Source: CAD feature listing. Evaluate the final solid. Frame: model axes, mm. A direction names the side the tool comes from. Coordinates: 2 decimals unless noted, no trailing zeros. Order: outer loops, then holes, each group sorted by start corner. A loop starts at its lowest first (then second) coordinate and runs counter-clockwise, first axis right, second up. Notation, with made-up numbers: (66.5, -33) -> (96.5, -33) arc R11 ccw to (96.5, -15) -> close; hole circle Ø5 at (11.5, 37.25). An arc over 180 degrees is marked (long way). Write each question's results on one line, items separated by ' | '. Start each with the question number.
from build123d import *

# Parameters (mm, degrees)
SKETCH1_W           = 13.208
SKETCH1_H           = 10.668
BOSS_EXTRUDE2_DEPTH = 10.16
SKETCH4_R           = 2.54
CUT_EXTRUDE1_DEPTH  = 38.1
SKETCH6_R           = 2.54
CUT_EXTRUDE2_DEPTH  = 10.16


with BuildPart() as part:
    # Sketch1 → Boss-Extrude2 (new body)
    with BuildSketch(Plane.XY):
        with BuildLine():
            Line((0, 0), (0, 66.04))
            ThreePointArc((0, 66.04), (1.487897552, 69.632102448), (5.08, 71.12))
            Line((5.08, 71.12), (33.02, 71.12))
            ThreePointArc((33.02, 71.12), (36.612102448, 69.632102448), (38.1, 66.04))
            Line((38.1, 66.04), (38.1, 0))
            Line((38.1, 0), (38.1, -5.08))
            ThreePointArc((38.1, -5.08), (36.612102448, -8.672102448), (33.02, -10.16))
            Line((33.02, -10.16), (5.08, -10.16))
            ThreePointArc((5.08, -10.16), (1.487897552, -8.672102448), (0, -5.08))
            Line((0, -5.08), (0, 0))
        make_face()
        with Locations((19.05, 5.334)):
            Rectangle(SKETCH1_W, SKETCH1_H, mode=Mode.SUBTRACT)
        with BuildLine():
            Line((9.525, 56.134), (9.525, 25.654))
            ThreePointArc((9.525, 25.654), (19.05, 16.129), (28.575, 25.654))
            Line((28.575, 25.654), (28.575, 56.134))
            ThreePointArc((28.575, 56.134), (19.05, 65.659), (9.525, 56.134))
        make_face(mode=Mode.SUBTRACT)
    extrude(amount=BOSS_EXTRUDE2_DEPTH)

    # Sketch4 → Cut-Extrude1 (cut)
    with BuildSketch(Plane.ZY):
        with Locations((5.08, 5.334)):
            Circle(SKETCH4_R)
    extrude(amount=-CUT_EXTRUDE1_DEPTH, mode=Mode.SUBTRACT)

    # Sketch6 → Cut-Extrude2 (cut)
    with BuildSketch(Plane.XZ.offset(10.16)):
        with Locations(Location((19.05, 5.08, 0), (0, 0, 270))):
            Circle(SKETCH6_R)
    extrude(amount=-CUT_EXTRUDE2_DEPTH, mode=Mode.SUBTRACT)


solid = part.part
(1) Section B-B on y = 41. Return the cut outline in (x, z) (3 decimals), then the cut area to 3 significant figures.
(2) Section D-D on x = 22.5. Return the cut outline in (y, z).
(3) Line query: L1, parallel to X at y = 33, z = 5 (3 decimals); L2, parallel to X at y = -2.5, z = 5.08; L3, parallel to Y at x = 14.5, z = 6.5. Output: solid intervals per line, ascending.
(4) Draft query along X for faces 3 (the flat face through (32, 31, 10.16)), 4 (the cylindrical face through (1.449, 69.592, 5.009)), 5 (the flat face through (9.525, 41, 5)), 6 (the cylindrical face through (16.57, -5.15, 5.63)). Return one class per face: released by +X, released by -X, zero draft, split by the parting line, or undercut.
(5) Section A-A on z = 5.08. Return the cut outline in (x, y) (3 decimals).
(6) Reachability of faces 1 (the flat face through (0, 30, 5)), 2 (the flat face through (19, 10.668, 5)) from +Z, -Z, +X, -X, +Y, -Y: full face, straight path, thin tool, end or side. Return the list, or none.
(7) Section C-C on z = 1.25. Return the cut outline in (x, y) (3 decimals).
(8) First-contact query: P1, Ø12, axis at x = 19.5, y = 37.5, coming from the -Z side. Flat tip, straight axial feed; report the tip coordinate or a pass-through.
Results list:
1) outline: (0, 0) -> (9.525, 0) -> (9.525, 10.16) -> (0, 10.16) -> close; (28.575, 0) -> (38.1, 0) -> (38.1, 10.16) -> (28.575, 10.16) -> close | area: 194 mm²
2) outline: (-10.16, 0) -> (0, 0) -> (0, 10.16) -> (-10.16, 10.16) -> close; (10.67, 0) -> (16.78, 0) -> (16.78, 10.16) -> (10.67, 10.16) -> close; (65.01, 0) -> (71.12, 0) -> (71.12, 10.16) -> (65.01, 10.16) -> close
3) L1: x = 0 to 9.525, 28.575 to 38.1 | L2: x = 0 to 16.51, 21.59 to 38.1 | L3: y = -10.16 to 0, 10.67 to 17.29, 64.5 to 71.12
4) face 3: zero draft | face 4: released by -X | face 5: undercut | face 6: undercut
5) outline: (0, -5.08) arc R5.08 ccw to (5.08, -10.16) -> (16.51, -10.16) -> (16.51, 0) -> (12.446, 0) -> (12.446, 2.794) -> (0, 2.794) -> close; (0, 7.874) -> (12.446, 7.874) -> (12.446, 10.668) -> (25.654, 10.668) -> (25.654, 7.874) -> (38.1, 7.874) -> (38.1, 66.04) arc R5.08 ccw to (33.02, 71.12) -> (5.08, 71.12) arc R5.08 ccw to (0, 66.04) -> close; (21.59, -10.16) -> (33.02, -10.16) arc R5.08 ccw to (38.1, -5.08) -> (38.1, 2.794) -> (25.654, 2.794) -> (25.654, 0) -> (21.59, 0) -> close; hole (9.525, 25.654) arc R9.525 ccw to (28.575, 25.654) -> (28.575, 56.134) arc R9.525 ccw to (9.525, 56.134) -> close
6) face 1: +Z, -Z, -X, +Y, -Y | face 2: +Z, -Z
7) outline: (0, -5.08) arc R5.08 ccw to (5.08, -10.16) -> (33.02, -10.16) arc R5.08 ccw to (38.1, -5.08) -> (38.1, 66.04) arc R5.08 ccw to (33.02, 71.12) -> (5.08, 71.12) arc R5.08 ccw to (0, 66.04) -> close; hole (9.525, 25.654) arc R9.525 ccw to (28.575, 25.654) -> (28.575, 56.134) arc R9.525 ccw to (9.525, 56.134) -> close; hole (12.446, 0) -> (25.654, 0) -> (25.654, 10.668) -> (12.446, 10.668) -> close
8) P1: passes through
